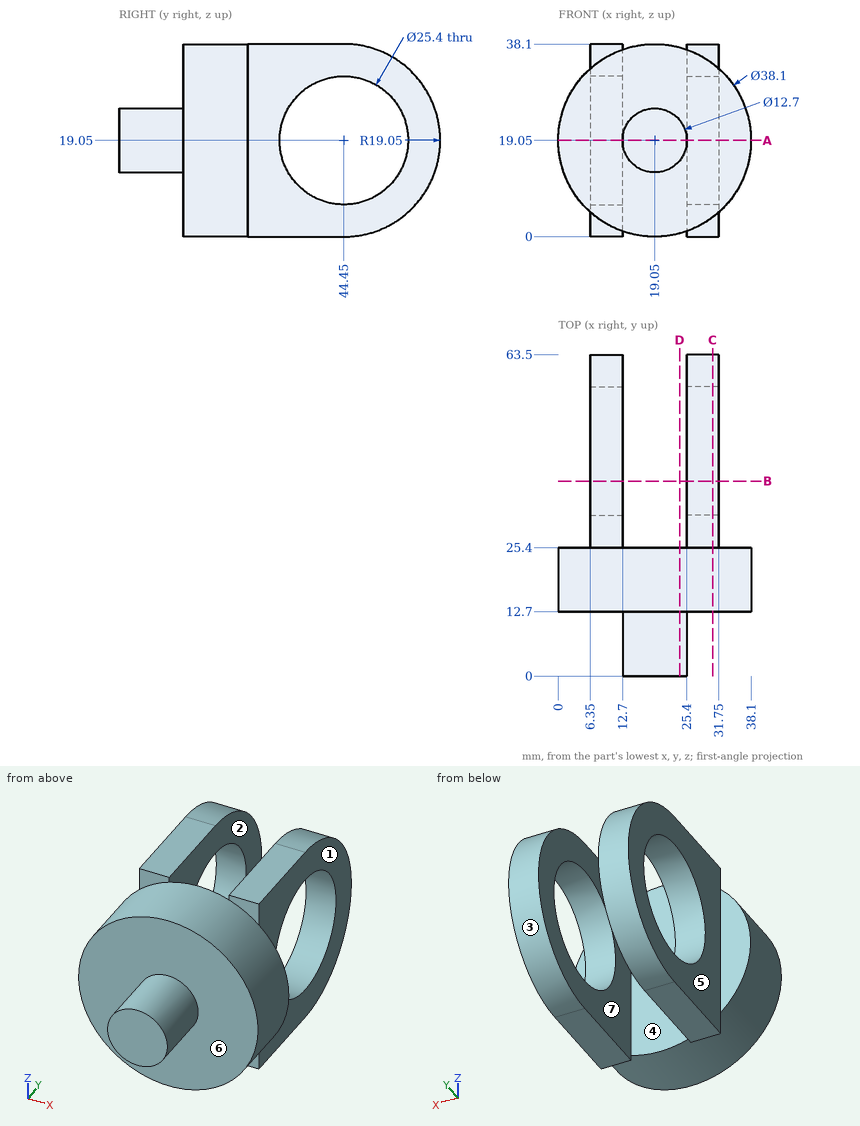
Could you check a few things on this drawing? It's one solid part, dimensions in mm from its lowest x, y, z. A direction names the side the tool comes from. Coordinates: 2 decimals unless noted, no trailing zeros. Order: outer loops, then holes, each group sorted by start corner. A loop starts at its lowest first (then second) coordinate and runs counter-clockwise, first axis right, second up. Notation, with made-up numbers: M -39.75,19.25 L -2.75,19.25 A14 ccw -2.75,31.25 Z; hole C -31,39 d10. An arc over 180 degrees is marked long. Use a Markdown table: item, result. Add a question column.
Q1. I want a section at C-C on x = 30.5. List the corners of the cut face in (y, z) for me, then the cut area to 3 significant figures.
Q2. I want a section at B-B on y = 38.5. List the corners of the cut face in (x, z) for me, then the cut area to 3 significant figures.
Q3. I want a section at A-A on z = 19.05. List the corners of the cut face in (x, y) for me.
Q4. I'm going to push flat-ended pins straight in: pin 1 (10 mm diameter, centred on y = 7.5, z = 21.5, fed in from +X); pin 2 (3 mm diameter, centred on x = 4.5, z = 7, fed in from +Y); pin 3 (2.5 mm diameter, centred on x = 27, z = 37, fed in from -Y); pin 4 (1 mm diameter, centred on y = 56, z = 19, fed in from +X). Where does each tip first touch, or does it pass through?
Q5. I want a section at D-D on x = 24. List the corners of the cut face in (y, z) for me.
Q6. We'd pull the mould along X, two halves only. Please class the marked faces 1, 2, 3 and 4: pulls with the +X half, pulls with the -X half, needs draft (parallel to the pull), parting line crosses it, or undercut.
Q7. Which directions (+Z, -Z, +X, -X, +Y, -Y) give clear straight access to the entire face, cutting with the end or side of a thin tool? Please do the marked faces 5, 6 and 7.
Q8. If I drill on L1, parallel to X at y = 31.5, z = 15; L2, parallel to Y at x = 9, z = 19.05; L3, parallel to Y at x = 5.5, z = 28.5, over which ranges is the centre line in solid material (lowest first)?
Checked values:
| question | item | result |
|---|---|---|
| 1 | outline | M 12.7,3.83 L 25.4,3.83 L 25.4,0 L 44.45,0 A19.05 ccw 44.45,38.1 L 25.4,38.1 L 25.4,34.27 L 12.7,34.27 Z; hole C 44.45,19.05 d25.4 |
| 1 | area | 1,180 mm² |
| 2 | outline | M 6.35,0 L 12.7,0 L 12.7,7.83 L 6.35,7.83 Z; M 6.35,30.27 L 12.7,30.27 L 12.7,38.1 L 6.35,38.1 Z; M 25.4,0 L 31.75,0 L 31.75,7.83 L 25.4,7.83 Z; M 25.4,30.27 L 31.75,30.27 L 31.75,38.1 L 25.4,38.1 Z |
| 2 | area | 199 mm² |
| 3 | outline | M 0,12.7 L 12.7,12.7 L 12.7,0 L 25.4,0 L 25.4,12.7 L 38.1,12.7 L 38.1,25.4 L 31.75,25.4 L 31.75,31.75 L 25.4,31.75 L 25.4,25.4 L 12.7,25.4 L 12.7,31.75 L 6.35,31.75 L 6.35,25.4 L 0,25.4 Z; M 6.35,57.15 L 12.7,57.15 L 12.7,63.5 L 6.35,63.5 Z; M 25.4,57.15 L 31.75,57.15 L 31.75,63.5 L 25.4,63.5 Z |
| 4 | pin 1 | x = 25.4 |
| 4 | pin 2 | y = 25.4 |
| 4 | pin 3 | y = 12.7 |
| 4 | pin 4 | through |
| 5 | outline | M 0,15.07 L 12.7,15.07 L 12.7,0.65 L 25.4,0.65 L 25.4,37.45 L 12.7,37.45 L 12.7,23.03 L 0,23.03 Z |
| 6 | face 1 | pulls with the +X half |
| 6 | face 2 | undercut |
| 6 | face 3 | needs draft |
| 6 | face 4 | undercut |
| 7 | face 5 | +Z, -Z, -X, +Y |
| 7 | face 6 | -Y |
| 7 | face 7 | +Z, -Z, +Y |
| 8 | L1 | 6.35 to 12.7, 25.4 to 31.75 |
| 8 | L2 | 12.7 to 31.75, 57.15 to 63.5 |
| 8 | L3 | 12.7 to 25.4 |
